Answer from the drawing. Dimensions are ordinates in mm from the lowest x, y and z of the part. Coordinates: 2 decimals unless noted, no trailing zeros. Order: outer loops, then holes, each group sorted by start corner. A loop starts at its lowest first (then second) coordinate and runs counter-clockwise, first axis right, second up. Notation, with made-up numbers: (79, -23) -> (84, -23) arc R21 ccw to (84, 4) -> close; hole circle Ø8 at (-7, 60). An arc over 180 degrees is marked (long way). Answer in a Markdown table with one row per item.
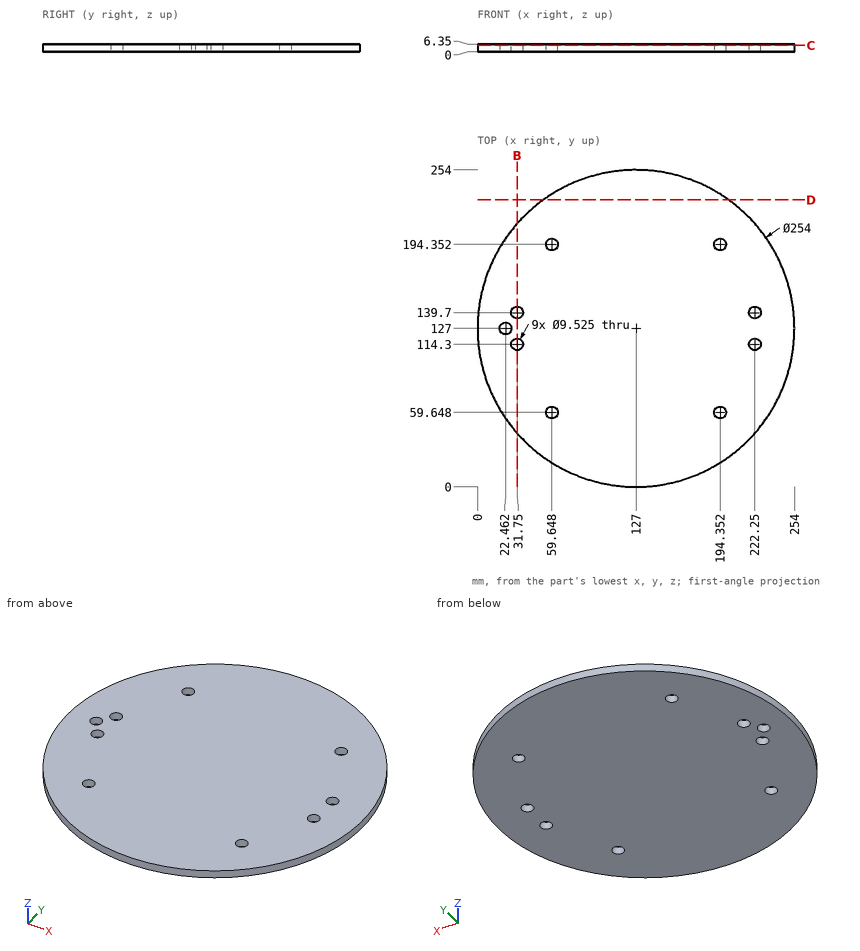
(1) Find the intervals of material crossed by line 1 along Y through (x, z) = (58.5, 3.75) (1 decimal); line 2 along Y through (x, z) = (222.25, 2.25) (1 decimal); line 3 along X through (y, z) = (139.7, 3.5), in increasing order. Write a range as from..to.
Check values:
| item | result |
|---|---|
| line 1 | 20.1..55, 64.3..189.7, 199..233.9 |
| line 2 | 43..109.5, 119.1..134.9, 144.5..211 |
| line 3 | 0.64..26.99, 36.51..217.49, 227.01..253.36 |
(2) A cutting plane is placed at D-D, the plane y = 230. Determine the outline of the cut face in (x, z).
Check values:
| item | result |
|---|---|
| outline | (52.7, 0) -> (201.3, 0) -> (201.3, 6.35) -> (52.7, 6.35) -> close |
(3) Flat-ended cylindrical pins translate along their axes: pin 1 (2 mm diameter, centred on x = 38, z = 4.5, fed in from -Y); pin 2 (3 mm diameter, centred on y = 136.5, z = 4, fed in from -X); pin 3 (8.5 mm diameter, centred on x = 31.75, y = 114.3, fed in from +Z); pin 4 (1.5 mm diameter, centred on y = 175.5, z = 4, fed in from -X). Find the tip coordinate at first contact, or state that the pin passes through.
Check values:
| item | result |
|---|---|
| pin 1 | y = 35.43 |
| pin 2 | x = 0.25 |
| pin 3 | through |
| pin 4 | x = 9.32 |
(4) A cutting plane is placed at B-B, the plane x = 31.75. Determine the outline of the cut face in (y, z).
Check values:
| item | result |
|---|---|
| outline | (43, 0) -> (109.54, 0) -> (109.54, 6.35) -> (43, 6.35) -> close; (119.06, 0) -> (134.94, 0) -> (134.94, 6.35) -> (119.06, 6.35) -> close; (144.46, 0) -> (211, 0) -> (211, 6.35) -> (144.46, 6.35) -> close |
(5) A cutting plane is placed at C-C, the plane z = 5.25. Count the separate pieces of the cut face and the enclosed holes in it, then the cut area to 3 significant figures.
Check values:
| item | result |
|---|---|
| separate pieces | 1 |
| enclosed holes | 9 |
| area | 50,000 mm² |
